Verification items for the finished model (mm, model axes). Face numbers are marked on the shaded views. A direction names the side the tool comes from. Give positions to 0.01 mm unless a question says otherwise; leave off trailing zeros. Order: outer loops, then holes, each group sorted by start corner. A loop starts at its lowest first (then second) coordinate and runs counter-clockwise, first axis right, second up. Notation, with made-up numbers: (22, 83) -> (71, 83) arc R12 ccw to (71, 102) -> close; hole circle Ø3 at (53, -20.5). An arc over 180 degrees is marked (long way). Return JSON: item names as keys, results as strings. Group by question number.
(1) Cross-section at D-D on z = 8.25. Enter the section's corners in (x, y), then the cut area to 3 significant figures.
(2) Cross-section at B-B on x = -30. Enter the section's corners in (y, z).
(3) Thickness scan on line 1 along X through (y, z) = (-9.3, 5); line 2 along X through (y, z) = (7.25, 8); line 3 along Y through (x, z) = (-18.5, 4.75). Record the ranges inside material, lowest first.
(4) Depth check by flat-ended pin: pin 1 Ø1.5 at (y, z) = (3.5, 8) entering from +X; pin 2 Ø5 at (x, y) = (-52.5, 5.5) entering from -Z; pin 3 Ø2.5 at (y, z) = (1.5, 8) entering from -X. Enter the tip coordinate at first touch or a pass-through.
(5) Cross-section at A-A on z = 5. Enter the section's corners in (x, y), then the cut area to 3 significant figures.
(6) Cross-section at C-C on y = 7.75. Enter the section's corners in (x, z).
(7) Tool access check on the marked faces 1 and 2. Record the directions out of +Z, -Z, +X, -X, +Y, -Y that give a thin tool (end or side, any length) a straight path to the whole face; none if there is none.
from build123d import *

# Parameters (mm, degrees)
SKETCH1_W               = 170
SKETCH1_H               = 3
BOSS_EXTRUDE1_DEPTH     = 10
SKETCH4_R               = 1.2
CUT_EXTRUDE1_DEPTH      = 21
SKETCH2_W               = 45.3
SKETCH2_H               = 3
BOSS_EXTRUDE6_DEPTH     = 20.3
SKETCH5_R               = 8.5
CUT_EXTRUDE2_DEPTH      = 20.3
SKETCH6_W               = 45.3
SKETCH6_H               = 3
BOSS_EXTRUDE7_DEPTH     = 20.3
SKETCH7_R               = 8.5
CUT_EXTRUDE3_DEPTH      = 100.885733504
CUT_EXTRUDE5_DEPTH      = 102.201856693
CUT_EXTRUDE5_DEPTH_BACK = 102.201856693
SKETCH12_W              = 88.7
SKETCH12_H              = 17.241657791
CUT_EXTRUDE6_DEPTH      = 75.862735481
CUT_EXTRUDE6_DEPTH_BACK = 75.862735481
SKETCH13_W              = 37.135878318
SKETCH13_H              = 38.462159687
SKETCH13_W_2            = 38.462159687
SKETCH13_H_2            = 47.746129266
SKETCH15_W              = 8
SKETCH15_H              = 10
BOSS_EXTRUDE9_DEPTH     = 3
CUT_EXTRUDE7_DEPTH      = 67.392895801
CUT_EXTRUDE7_DEPTH_BACK = 67.392895801
SKETCH16_R              = 1.5


with BuildPart() as part:
    # Sketch1 → Boss-Extrude1 (new body)
    with BuildSketch(Plane.XY):
        with Locations((13.639372454, -9.657761352)):
            Rectangle(SKETCH1_W, SKETCH1_H)
    extrude(amount=BOSS_EXTRUDE1_DEPTH)

    # Sketch4 → Cut-Extrude1 (cut)
    with BuildSketch(Plane(origin=(0, -8.157761352, 0), x_dir=(1, 0, 0), z_dir=(0, 1, 0))):
        with Locations(Location((-63.360627546, -4.938536908, 0), (0, 0, 180))):
            Circle(SKETCH4_R)
        with Locations(Location((90.639372454, -5.283238547, 0), (0, 0, 180))):
            Circle(SKETCH4_R)
    extrude(amount=-CUT_EXTRUDE1_DEPTH, mode=Mode.SUBTRACT)

    # Sketch2 → Boss-Extrude6 (add)
    with BuildSketch(Plane(origin=(0, -8.157761352, 0), x_dir=(1, 0, 0), z_dir=(0, 1, 0))):
        with Locations((-30.710627546, -8.5)):
            Rectangle(SKETCH2_W, SKETCH2_H)
    extrude(amount=BOSS_EXTRUDE6_DEPTH)

    # Sketch5 → Cut-Extrude2 (cut)
    with BuildSketch(Plane(origin=(0, 0, 7), x_dir=(-1, 0, 0), z_dir=(0, 0, -1))):
        with Locations((17.460627546, 1.942238648)):
            Circle(SKETCH5_R)
        with Locations((43.960627546, 1.942238648)):
            Circle(SKETCH5_R)
        with BuildLine():
            Line((27.510627546, -3.557761352), (33.910627546, -3.557761352))
            ThreePointArc((33.910627546, -3.557761352), (35.810627546, -5.457761352), (33.910627546, -7.357761352))
            Line((33.910627546, -7.357761352), (27.510627546, -7.357761352))
            ThreePointArc((27.510627546, -7.357761352), (25.610627546, -5.457761352), (27.510627546, -3.557761352))
        make_face()
    extrude(amount=-CUT_EXTRUDE2_DEPTH, mode=Mode.SUBTRACT)

    # Sketch6 → Boss-Extrude7 (add)
    with BuildSketch(Plane(origin=(0, -8.157761352, 0), x_dir=(1, 0, 0), z_dir=(0, 1, 0))):
        with Locations((57.989372454, -8.5)):
            Rectangle(SKETCH6_W, SKETCH6_H)
    extrude(amount=BOSS_EXTRUDE7_DEPTH)

    # Sketch7 → Cut-Extrude3 (cut, through all)
    with BuildSketch(Plane.XY.offset(10)):
        with Locations((44.739372454, 1.942238648)):
            Circle(SKETCH7_R)
        with Locations((71.239372454, 1.942238648)):
            Circle(SKETCH7_R)
        with BuildLine():
            Line((54.839372454, -3.557761352), (61.239372454, -3.557761352))
            ThreePointArc((61.239372454, -3.557761352), (63.139372454, -5.457761352), (61.239372454, -7.357761352))
            Line((61.239372454, -7.357761352), (54.839372454, -7.357761352))
            ThreePointArc((54.839372454, -7.357761352), (52.939372454, -5.457761352), (54.839372454, -3.557761352))
        make_face()
    extrude(amount=-CUT_EXTRUDE3_DEPTH, mode=Mode.SUBTRACT)

    # Sketch12 → Cut-Extrude5 (cut, two sides: drawn at the far end of the back side and taken through both)
    with BuildSketch(Plane(origin=(0, -8.157761352, 0), x_dir=(1, 0, 0), z_dir=(0, 1, 0)).offset(-CUT_EXTRUDE5_DEPTH_BACK)):
        with Locations((54.289372454, -4.61843826)):
            Rectangle(SKETCH12_W, SKETCH12_H)
    extrude(amount=CUT_EXTRUDE5_DEPTH + CUT_EXTRUDE5_DEPTH_BACK, mode=Mode.SUBTRACT)

    # Sketch13 → Cut-Extrude6 (cut, two sides: drawn at the far end of the back side and taken through both)
    with BuildSketch(Plane(origin=(0, -8.157761352, 0), x_dir=(1, 0, 0), z_dir=(0, 1, 0)).offset(-CUT_EXTRUDE6_DEPTH_BACK)):
        with Locations((-71.928566705, 3.983905185)):
            Rectangle(SKETCH13_W, SKETCH13_H)
        with Locations((11.170452297, -17.070811541)):
            Rectangle(SKETCH13_W_2, SKETCH13_H_2)
    extrude(amount=CUT_EXTRUDE6_DEPTH + CUT_EXTRUDE6_DEPTH_BACK, mode=Mode.SUBTRACT)

    # Sketch15 → Boss-Extrude9 (add)
    with BuildSketch(Plane.XZ.offset(11.157761352)):
        with Locations((-57.360627546, 5)):
            Rectangle(SKETCH15_W, SKETCH15_H)
        with Locations((-4.060627546, 5)):
            Rectangle(SKETCH15_W, SKETCH15_H)
    extrude(amount=-BOSS_EXTRUDE9_DEPTH)

    # Sketch16 → Cut-Extrude7 (cut, two sides: drawn at the far end of the back side and taken through both)
    with BuildSketch(Plane(origin=(0, -11.157761352, 0), x_dir=(-1, 0, 0), z_dir=(0, -1, 0)).offset(-CUT_EXTRUDE7_DEPTH_BACK)):
        with Locations(Location((57.360627546, -5, 0), (0, 0, 180))):
            Circle(SKETCH16_R)
        with Locations(Location((4.060627546, -5, 0), (0, 0, 180))):
            Circle(SKETCH16_R)
    extrude(amount=CUT_EXTRUDE7_DEPTH + CUT_EXTRUDE7_DEPTH_BACK, mode=Mode.SUBTRACT)


solid = part.part
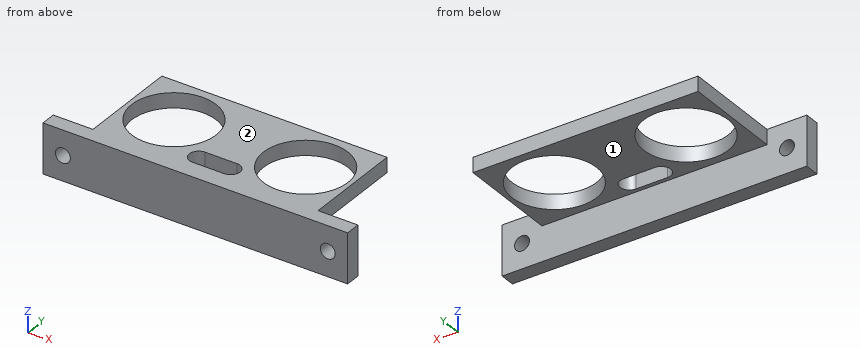
Verdict:
{
 "1": {"outline": "(-61.36, -11.16) -> (-0.06, -11.16) -> (-0.06, -8.16) -> (-8.06, -8.16) -> (-8.06, 12.14) -> (-53.36, 12.14) -> (-53.36, -8.16) -> (-61.36, -8.16) -> close; hole circle Ø17 at (-43.96, 1.94); hole (-33.91, -7.36) -> (-27.51, -7.36) arc R1.9 ccw to (-27.51, -3.56) -> (-33.91, -3.56) arc R1.9 ccw to start; hole circle Ø17 at (-17.46, 1.94)", "area": "614 mm²"},
 "2": {"outline": "(-11.16, 0) -> (-8.16, 0) -> (-8.16, 7) -> (-7.36, 7) -> (-7.36, 10) -> (-11.16, 10) -> close; (-3.56, 7) -> (12.14, 7) -> (12.14, 10) -> (-3.56, 10) -> close"},
 "3": {"line 1": "-61.36 to -58.86, -55.86 to -5.56, -2.56 to -0.06", "line 2": "-53.36 to -50.6, -37.32 to -24.1, -10.82 to -8.06", "line 3": "-11.16 to -8.16"},
 "4": {"pin 1": "x = -8.06", "pin 2": "z = 7", "pin 3": "x = -53.36"},
 "5": {"outline": "(-61.36, -11.16) -> (-58.86, -11.16) -> (-58.86, -8.16) -> (-61.36, -8.16) -> close; (-55.86, -11.16) -> (-5.56, -11.16) -> (-5.56, -8.16) -> (-55.86, -8.16) -> close; (-2.56, -11.16) -> (-0.06, -11.16) -> (-0.06, -8.16) -> (-2.56, -8.16) -> close", "area": "166 mm²"},
 "6": {"outline": "(-53.36, 7) -> (-50.17, 7) -> (-50.17, 10) -> (-53.36, 10) -> close; (-37.75, 7) -> (-23.67, 7) -> (-23.67, 10) -> (-37.75, 10) -> close; (-11.25, 7) -> (-8.06, 7) -> (-8.06, 10) -> (-11.25, 10) -> close"},
 "7": {"face 1": "-Z, +X, -X, +Y", "face 2": "+Z, +X, -X, +Y, -Y"}
}
